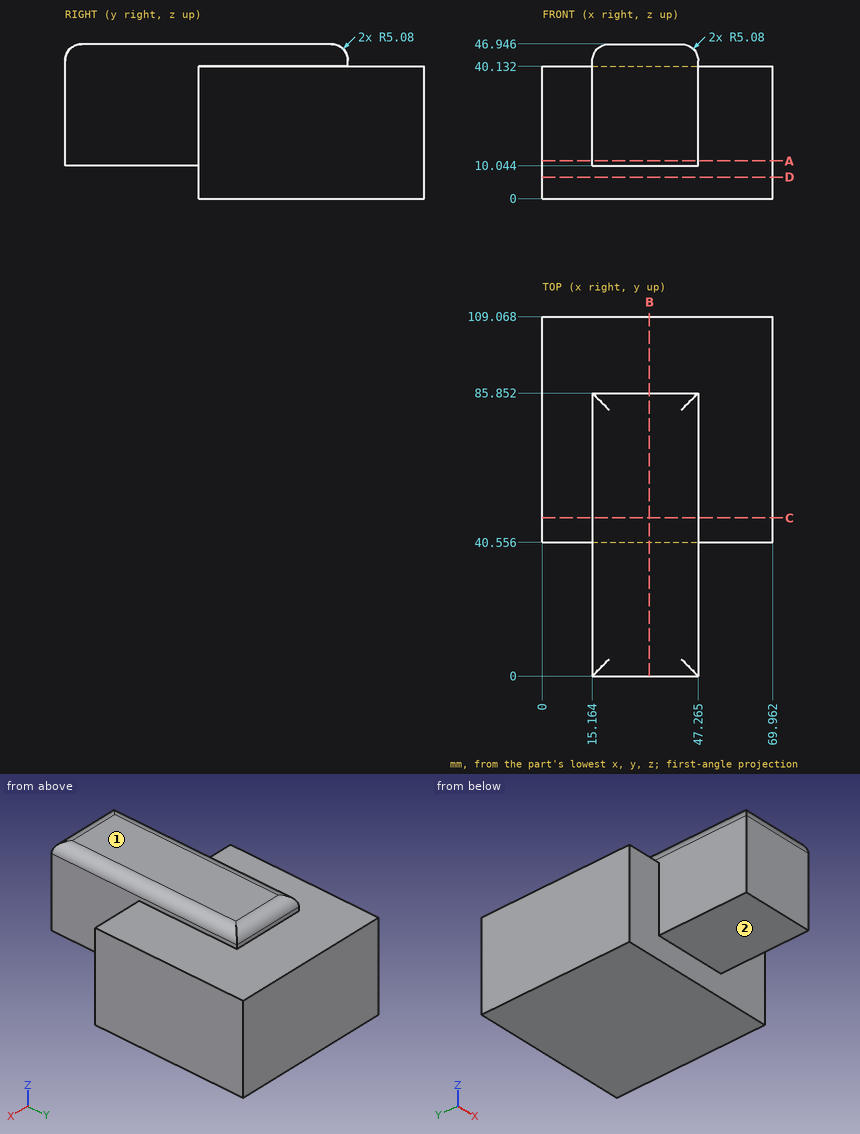
Print and shaded views of the part. All mm, measured from the part's lowest x, y and z. A direction names the side the tool comes from. Give positions to 0.01 mm unless a question says otherwise; leave off trailing zeros. Loops run counter-clockwise (first coordinate to the right, second up) from the corner with the lowest first, then second, coordinate; pieces in that order, holes last.
1) Wall check: line 1 (Z direction, x = 57.5, y = 73); line 2 (Y direction, x = 34.5, z = 8); line 3 (Z direction, x = 38, y = 36) (1 decimal). Give the ranges that are in metal, low to high.
2) Saw through at A-A (z = 11.5). Write the cut outline in (x, y) (1 decimal), plus the area to 4 significant figures.
3) Tool access for the marked faces 1 and 2: list every direction of +Z, -Z, +X, -X, +Y, -Y with a clear straight run to the whole face (end or side of a thin tool).
4) Flat gauge pins, fed straight in: pin 1 Ø8 at (x, z) = (48.5, 6) entering from -Y; pin 2 Ø0.5 at (x, z) = (31.5, 40.5) entering from +Y; pin 3 Ø12 at (x, y) = (49.5, 20) entering from +Z. Where does each tip first touch, or does it go through?
5) Saw through at B-B (x = 32.5). Write the cut outline in (y, z) (1 decimal), plus the area to 3 significant figures.
6) Saw through at D-D (z = 6.5). Write the cut outline in (x, y), plus the area to 3 significant figures.
7) Saw through at C-C (y = 48). Write the cut outline in (x, z) (1 decimal), plus the area to 3 significant figures.
Answer block:
1. line 1: z = 0 to 40.13
1. line 2: y = 40.56 to 109.07
1. line 3: z = 10 to 46.9
2. outline: (0, 40.6) - (15.2, 40.6) - (15.2, 0) - (47.3, 0) - (47.3, 40.6) - (70, 40.6) - (70, 109.1) - (0, 109.1) - close
2. area: 6,095 mm2
3. face 1: +Z, +X, -X, +Y, -Y
3. face 2: -Z, +X, -X, -Y
4. pin 1: stops at y = 40.56
4. pin 2: stops at y = 85.85
4. pin 3: stops at z = 46.77
5. outline: (0, 10) - (40.6, 10) - (40.6, 0) - (109.1, 0) - (109.1, 40.1) - (85.9, 40.1) - (85.9, 41.9) arc R5.1 ccw to (80.8, 46.9) - (5.1, 46.9) arc R5.1 ccw to (0, 41.9) - close
5. area: 4,540 mm2
6. outline: (0, 40.56) - (69.96, 40.56) - (69.96, 109.07) - (0, 109.07) - close
6. area: 4,790 mm2
7. outline: (0, 0) - (70, 0) - (70, 40.1) - (47.3, 40.1) - (47.3, 41.9) arc R5.1 ccw to (42.2, 46.9) - (20.2, 46.9) arc R5.1 ccw to (15.2, 41.9) - (15.2, 40.1) - (0, 40.1) - close
7. area: 3,020 mm2
